Design review of the part built by this model. Coordinates are the model's own, in mm. Face numbers are marked on the shaded views. A direction names the side the tool comes from. Coordinates: 2 decimals unless noted, no trailing zeros. Write each loop counter-clockwise with the first axis right and the second up, starting at its lowest first coordinate (ties: lowest second). Pieces come first, ordered by that corner, then holes. Notation, with made-up numbers: (45.5, 19.25) -> (70.5, 19.25) arc R19 cw to (70.5, 24.25) -> close; hole circle Ø6 at (-5, 23). An arc over 180 degrees is marked (long way). One line per question, with ' | ' between items. Start each with the question number.
Q1. Add section B-B on z = 28.5. State the section outline as (x, y) points.
Q2. Add section A-A on x = 44.5. State the section outline as (y, z) points.
Q3. Add section D-D on x = 27. State the section outline as (y, z) points, and give its area (3 significant figures).
Q4. Add section C-C on y = 2. State the section outline as (x, z) points, and give its area (3 significant figures).
Q5. Wall thickness on probe 1 along Y at (x, z) = (29, 8.5); probe 2 along Z at (x, y) = (29, 1); probe 3 along X at (y, z) = (7.75, 21.5): over which ranges is each line inside the solid? List them lowest first.
Q6. For the marked faces 1, 2 and 3, list the 3-axis set-ups (+Z, -Z, +X, -X, +Y, -Y) from which the entire face can be reached by the end or side of a thin tool; tool diameter is ignored.
Q7. For P1, Ø0.5, axis at x = 47.5, z = 29, coming from the +Y side; P2, Ø7, axis at x = 45.51, y = 5.21, coming from the -Z side; P3, Ø2, axis at y = 3.5, z = 37, coming from the +X side, all flat-tipped, find the tip position at first contact; note any pin that passes through.
Solid Edge part; units mm, degrees
sketch "Sketch1" plane through (0, 0, 0) normal (0, -1, 0) x (1, 0, 0)
  line L0 (0.6959, 36.2554) -> (0.6959, 0.7554)
  line L1 (0.6959, 0.7554) -> (41.1959, 0.7554)
  line L2 (41.1959, 36.2554) -> (41.1959, 0.7554)
  line L3 (0.6959, 36.2554) -> (41.1959, 36.2554)
  line L4 (-6.3041, 30.2554) -> (0.6959, 30.2554)
  line L5 (0.6959, 30.2554) -> (0.6959, 27.7554)
  line L6 (-6.3041, 27.7554) -> (0.6959, 27.7554)
  line L7 (-6.3041, 27.7554) -> (-6.3041, 30.2554)
  line L8 (48.1959, 27.7554) -> (41.1959, 27.7554)
  line L9 (41.1959, 30.2554) -> (41.1959, 27.7554)
  line L10 (48.1959, 30.2554) -> (41.1959, 30.2554)
  line L11 (48.1959, 27.7554) -> (48.1959, 30.2554)
extrude "Protrusion1" add sketch "Sketch1" against normal blind 20
sketch "Sketch2" plane through (-2.8041, 10, 30.2554) normal (0, 0, 1) x (1, 0, 0)
  line L0 (-3.5, 8.964) -> (3.5, 8.964)
  line L1 (3.5, 8.964) -> (3.5, 10.8897)
  line L2 (3.5, 10.8897) -> (-4.9405, 10.8897)
  line L3 (-4.9405, 10.8897) -> (-4.7039, -10.9349)
  line L4 (-4.7039, -10.9349) -> (3.5, -10.9349)
  line L5 (3.5, -10.9349) -> (3.5, -9.036)
  line L6 (3.5, -9.036) -> (-3.5, -9.036)
  line L7 (-3.5, -9.036) -> (-3.5, -6.286)
  line L8 (-3.5, -6.286) -> (-2.4891, -6.286)
  arc A0 (-2.4891, -6.286) -> (-2.4891, -3.286) centre (-0.812, -4.786) ccw
  line L9 (-2.4891, -3.286) -> (-3.5, -3.286)
  line L10 (-3.5, -3.286) -> (-3.5, 3.1474)
  line L11 (-3.5, 3.1474) -> (-2.4271, 3.1474)
  arc A1 (-2.4271, 3.1474) -> (-2.4271, 6.2806) centre (-0.812, 4.714) ccw
  line L12 (-2.4271, 6.2806) -> (-3.5, 6.2806)
  line L13 (-3.5, 6.2806) -> (-3.5, 8.964)
extrude "Cutout1" cut sketch "Sketch2" against normal up to vertex (2.5 mm away)
mirror "Mirror1" about plane through (20.9459, 10, 18.5054) normal (-1, 0, 0) of "Cutout1"
sketch "Sketch3" plane through (20.9459, 10, 36.2554) normal (0, 0, 1) x (1, 0, 0)
  arc A0 (-5.812, 8.964) -> (-5.812, -9.036) centre (-10.1709, -0.036) ccw
  line L0 (-5.812, -9.036) -> (14.188, -9.036)
  line L1 (14.188, -9.036) -> (14.188, -4.836)
  arc A1 (14.188, -4.836) -> (14.188, 4.764) centre (10.588, -0.036) ccw
  line L2 (14.188, 4.764) -> (14.188, 8.964)
  line L3 (14.188, 8.964) -> (-5.812, 8.964)
extrude "Protrusion2" add sketch "Sketch3" along normal up to vertex (2 mm away)
sketch "Sketch4" plane through (19.1544, 9.964, 38.2554) normal (0, 0, 1) x (1, 0, 0)
  circle A0 centre (-8.3794, 0) radius 6.4
extrude "Protrusion3" add sketch "Sketch4" along normal up to vertex (1 mm away)
sketch "Sketch5" plane through (10.775, 9.964, 39.2554) normal (0, 0, 1) x (1, 0, 0)
  circle A0 centre (0, 0) radius 5.575
extrude "Protrusion4" add sketch "Sketch5" along normal up to vertex (0.5 mm away)
sketch "Sketch6" plane through (10.775, 9.964, 39.7554) normal (0, 0, 1) x (1, 0, 0)
  circle A0 centre (0, 0) radius 2.95
extrude "Protrusion5" add sketch "Sketch6" along normal up to vertex (4 mm away)
sketch "Sketch7" plane through (10.775, 9.964, 43.7554) normal (0, 0, 1) x (1, 0, 0)
  circle A0 centre (0, 0) radius 1.15
extrude "Cutout3" cut sketch "Sketch7" against normal up to vertex (4 mm away)
sketch "Sketch8" plane through (20.9459, 0, 18.5054) normal (0, -1, 0) x (0, 0, 1)
  line L0 (17.75, 20.25) -> (-17.75, 20.25)
extrude "Enlèvement_matière_6" cut sketch "Sketch8" against normal blind 73.875 material side at (0.6459, 0, 18.5054)
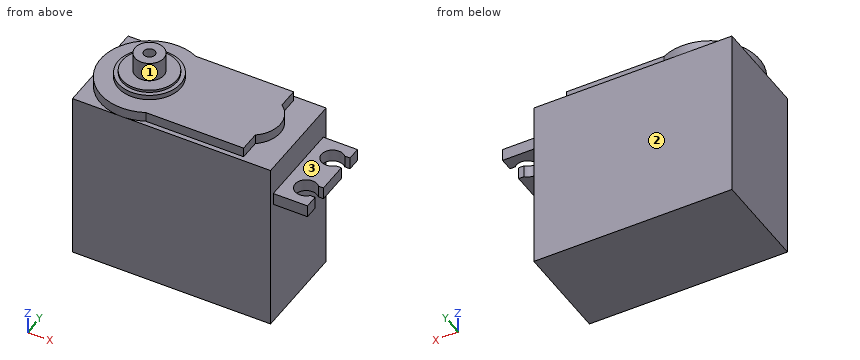
Output values:
1) outline: (0.7, 0) -> (41.2, 0) -> (41.2, 0.96) -> (48.2, 0.96) -> (48.2, 3.71) -> (47.18, 3.71) arc R2.25 cw (long way) to (47.18, 6.71) -> (48.2, 6.71) -> (48.2, 13.15) -> (47.12, 13.15) arc R2.25 cw (long way) to (47.12, 16.28) -> (48.2, 16.28) -> (48.2, 18.96) -> (41.2, 18.96) -> (41.2, 20) -> (0.7, 20) -> close
2) outline: (0.96, 27.76) -> (3.2, 27.76) -> (3.2, 30.26) -> (0.96, 30.26) -> close; (7.23, 27.76) -> (12.7, 27.76) -> (12.7, 30.26) -> (7.23, 30.26) -> close; (16.73, 27.76) -> (18.96, 27.76) -> (18.96, 30.26) -> (16.73, 30.26) -> close
3) outline: (0, 0.76) -> (20, 0.76) -> (20, 36.26) -> (18.96, 36.26) -> (18.96, 38.26) -> (0.96, 38.26) -> (0.96, 36.26) -> (0, 36.26) -> close | area: 746 mm2
4) outline: (0.7, 0.76) -> (41.2, 0.76) -> (41.2, 27.76) -> (48.2, 27.76) -> (48.2, 30.26) -> (41.2, 30.26) -> (41.2, 36.26) -> (35.13, 36.26) -> (35.13, 38.26) -> (4.73, 38.26) -> (4.73, 36.26) -> (0.7, 36.26) -> close | area: 1,520 mm2
5) probe 1: y = 0 to 20 | probe 2: z = 0.76 to 38.26 | probe 3: x = 0.7 to 41.2
6) face 1: +Z | face 2: +Z, -Z, +X, -X, +Y | face 3: +Z, +X, +Y, -Y
7) P1: stops at y = 18.96 | P2: stops at z = 27.76 | P3: stops at x = 41.2
